Geometry: final body of the model. Coordinates: model frame, mm. Give positions to 0.01 mm unless a question says otherwise; leave off trailing zeros. Write each loop counter-clockwise with the first axis right and the second up, starting at its lowest first coordinate (ties: lowest second). Pieces come first, ordered by that corner, then holes.
Q1. Section C-C (z = 3.25). Return the cut outline in (x, y), plus the area to 3 significant figures.
Q2. Pin query (flat end, axial travel): pin 1 Ø1.5 at (y, z) = (-4, 10) entering from -X; pin 2 Ø1 at (x, z) = (-14, 10) entering from +Y; pin 3 Ø1 at (y, z) = (9, 4.5) entering from +X. Return the tip coordinate at first contact, or that it passes through.
Q3. Line query: line 1 (Y direction, x = 0, z = 6.5); line 2 (X direction, y = -1, z = 1.25); line 3 (Y direction, x = -14, z = 1.75). Output: solid intervals per line, ascending.
Q4. Mould query, pull axis X, two halves, no side actions, for faces 1 (the cylindrical face through (-2.87, 2.64, 5.92)), 2 (the flat face through (3, -3, 0)). Classes: +X half, -X half, draft (parallel to the pull), parting line (faces both ways), or undercut.
Q5. Section D-D (z = 8.5). Return the cut outline in (x, y), plus the area to 3 significant figures.
from build123d import *

# Parameters (mm, degrees)
SKETCH_1_R      = 21.2
SKETCH_1_R_2    = 3.9
EXTRUDE_1_DEPTH = 12
FILLET_1_R      = 6
FILLET_2_R      = 6


with BuildPart() as part:
    # 草圖1 → 填料-伸長1 (new body)
    with BuildSketch(Plane.XY):
        Circle(SKETCH_1_R)
        Circle(SKETCH_1_R_2, mode=Mode.SUBTRACT)
    extrude(amount=EXTRUDE_1_DEPTH)

    # 圓角1
    fillet_1_edges = [part.edges().sort_by_distance(p)[0] for p in [
        (-21.2, 0, 12),
    ]]
    fillet(fillet_1_edges, radius=FILLET_1_R)

    # 圓角2
    fillet_2_edges = [part.edges().sort_by_distance(p)[0] for p in [
        (-21.2, 0, 0),
    ]]
    fillet(fillet_2_edges, radius=FILLET_2_R - 0.0001)  # a hair under: the kernel refuses the full size


solid = part.part
Computed:
1. outline: circle Ø41.07 at (0, 0); hole circle Ø7.8 at (0, 0)
1. area: 1,280 mm2
2. pin 1: stops at x = -19.87
2. pin 2: stops at y = 14.57
2. pin 3: stops at x = 19.25
3. line 1: y = -21.18 to -3.9, 3.9 to 21.18
3. line 2: x = -18.84 to -3.77, 3.77 to 18.84
3. line 3: y = -13.48 to 13.48
4. face 1: undercut
4. face 2: draft
5. outline: circle Ø41.31 at (0, 0); hole circle Ø7.8 at (0, 0)
5. area: 1,290 mm2
